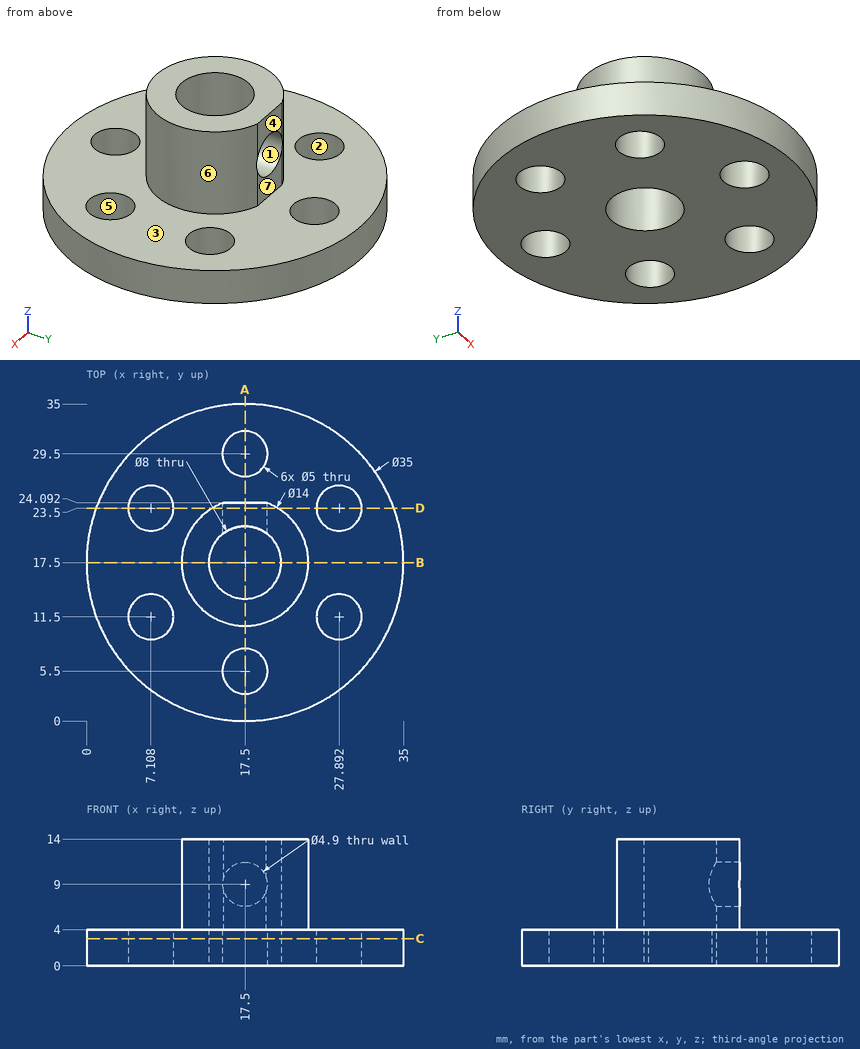
Design review of the part shown in the three views and the two pictorial views. Dimensions are in mm from the part's minimum x, y and z. A direction names the side the tool comes from. Round coordinates to 2 decimals unless told otherwise and drop trailing zeros. Write each loop counter-clockwise with the first axis right and the second up, starting at its lowest first coordinate (ties: lowest second). Pieces come first, ordered by that corner, then holes. Notation, with made-up numbers: (-32.5, 37.5) -> (9.5, 37.5) arc R18 ccw to (9.5, 56.5) -> close; hole circle Ø10 at (33.25, 2). An arc over 180 degrees is marked (long way). Answer as a JSON object with one key per item and string values.
1. We need section C-C on z = 3. State the section outline as (x, y) points.
Results found:
{"outline": "circle Ø35 at (17.5, 17.5); hole circle Ø5 at (7.11, 11.5); hole circle Ø5 at (7.11, 23.5); hole circle Ø8 at (17.5, 17.5); hole circle Ø5 at (17.5, 5.5); hole circle Ø5 at (17.5, 29.5); hole circle Ø5 at (27.89, 11.5); hole circle Ø5 at (27.89, 23.5)"}
2. Machinability: for the marked faces 1, 2, 3 and 4, which of the approach directions +Z, -Z, +X, -X, +Y, -Y give a long, thin tool a straight path to every point of the face, cutting with its end or side? Answer none if there is none.
Results found:
{"face 1": "+Y", "face 2": "+Z, -Z", "face 3": "+Z", "face 4": "+Z, +X, -X, +Y"}
3. We need section D-D on y = 23.5. State how many separate pieces and enclosed holes the cut face has, and give its area (3 significant figures).
Results found:
{"separate pieces": "3", "enclosed holes": "1", "area": "145 mm^2"}
4. We need section B-B on y = 17.5. State the section outline as (x, z) points, and give its area (3 significant figures).
Results found:
{"outline": "(0, 0) -> (13.5, 0) -> (13.5, 14) -> (10.5, 14) -> (10.5, 4) -> (0, 4) -> close; (21.5, 0) -> (35, 0) -> (35, 4) -> (24.5, 4) -> (24.5, 14) -> (21.5, 14) -> close", "area": "168 mm^2"}
5. The part is to be moulded in two halves that separate along Y. For the marked faces 5, 6 and 7, say which applies: pulls with the +Y half, pulls with the -Y half, needs draft (parallel to the pull), parting line crosses it, or undercut.
Results found:
{"face 5": "undercut", "face 6": "parting line crosses it", "face 7": "pulls with the +Y half"}
6. We need section A-A on x = 17.5. State the section outline as (y, z) points, and give its area (3 significant figures).
Results found:
{"outline": "(0, 0) -> (3, 0) -> (3, 4) -> (0, 4) -> close; (8, 0) -> (13.5, 0) -> (13.5, 14) -> (10.5, 14) -> (10.5, 4) -> (8, 4) -> close; (21.5, 0) -> (27, 0) -> (27, 4) -> (24.09, 4) -> (24.09, 6.55) -> (21.5, 6.55) -> close; (21.5, 11.45) -> (24.09, 11.45) -> (24.09, 14) -> (21.5, 14) -> close; (32, 0) -> (35, 0) -> (35, 4) -> (32, 4) -> close", "area": "111 mm^2"}
7. To check wall thickness, follow line 1 along Y through (x, z) = (17.5, 2.65); line 2 along Z through (x, y) = (5, 10); line 3 along Y through (x, z) = (17.5, 11). State the ranges of each line that lie inside material, in increasing order.
Results found:
{"line 1": "y = 0 to 3, 8 to 13.5, 21.5 to 27, 32 to 35", "line 2": "z = 0 to 4", "line 3": "y = 10.5 to 13.5"}
8. Clearance check with flat-ended pins moving along their axes: pin 1 (4.5 mm diameter, centred on x = 17.5, z = 9, fed in from -Y); pin 2 (3 mm diameter, centred on x = 27.89, y = 23.5, fed in from -Z); pin 3 (5 mm diameter, centred on x = 18, z = 12, fed in from +Y); pin 4 (5 mm diameter, centred on x = 21, z = 4, fed in from -Y). State where each tip first meets the part, or that it passes through.
Results found:
{"pin 1": "stops at y = 10.5", "pin 2": "passes through", "pin 3": "stops at y = 24.09", "pin 4": "stops at y = 0.03"}
